Part model, mm, in its own coordinate system. A direction names the side the tool comes from. Round coordinates to 2 decimals unless told otherwise and drop trailing zeros. Loops run counter-clockwise (first coordinate to the right, second up) from the corner with the lowest first, then second, coordinate; pieces in that order, holes last.
1) Band-saw the part on A-A, the plane z = 30.5. Write the cut outline in (x, y), then the cut area to 3 significant figures.
2) Probe line 1 (Y direction, x = 13.5, z = 8.5); line 2 (X direction, y = 0, z = 29.7). List the from-to ranges inside material, lowest first.
3) Drop flat-ended pins along their axis: P1, Ø2, axis at x = 12, y = 3.5, coming from the -Z side; P2, Ø11.5, axis at x = 0, y = 0, coming from the -Z side; P3, Ø1.5, axis at x = -11.5, y = -6.5, coming from the +Z side; P4, Ø1.5, axis at x = -13.5, y = -0.5, coming from the +Z side. Give the stop position or say it passes through.
4) Mould opens along X. For faces 1 (the cylindrical face through (8.89, -16.01, 12.62)), 2 (the conical face through (8.17, -8.33, 32.24)), 3 (the flat face through (8, -7, 33.5)) say: +X half, -X half, draft (parallel to the pull), parting line (faces both ways), or undercut.
5) Band-saw the part on B-B, the plane y = 0. Write the cut outline in (x, z), then the cut area to 3 significant figures.
6) Band-saw the part on D-D, the plane z = 13. Write the cut outline in (x, y).
7) Band-saw the part on C-C, the plane z = 2. Write the cut outline in (x, y), then the cut area to 3 significant figures.
8) 3-axis set-ups, long thin cutter, end or side, ignore diameter. For faces 4 (the cylindrical face through (-7.406, -16.014, 13.875)), 5 (the cylindrical face through (8.21, 8.05, 30.99)), 6 (the cylindrical face through (8.05, -8.21, 30.99)): which of +Z, -Z, +X, -X, +Y, -Y reach the whole face in a straight line?
from build123d import *

# Parameters (mm, degrees)
F0_W      = 34
F0_H      = 34
F0_W_2    = 30
F0_H_2    = 30
F1_DEPTH  = 2
F2_DEPTH  = 28
F4_W      = 34
F4_H      = 34
F4_W_2    = 30
F4_H_2    = 30
F5_DEPTH  = 2
F9_DEPTH  = 3.5
F3_R      = 4.05
F3_R_2    = 1
F3_R_3    = 1.0373308001
F10_DEPTH = 2
F11_W     = 34
F11_H     = 34
F12_DEPTH = 2


with BuildPart() as f1:
    # F0 (on Top) → F1 (new body)
    with BuildSketch(Plane.XY):
        Rectangle(F0_W, F0_H)
        Rectangle(F0_W_2, F0_H_2, mode=Mode.SUBTRACT)
        Rectangle(F0_W_2, F0_H_2)
    extrude(amount=-F1_DEPTH)

    # F0 (on Top) → F2 (join)
    with BuildSketch(Plane.XY):
        Rectangle(F0_W, F0_H)
        Rectangle(F0_W_2, F0_H_2, mode=Mode.SUBTRACT)
    extrude(amount=F2_DEPTH)

    # F4 (on face) → F5 (join)
    with BuildSketch(Plane.XY.offset(28)):
        Rectangle(F4_W, F4_H)
        Rectangle(F4_W_2, F4_H_2, mode=Mode.SUBTRACT)
        Rectangle(F4_W_2, F4_H_2)
        with BuildLine():
            ThreePointArc((11.4562390281, 1.0022910416), (11.4890545482, 0.5016229547), (11.5, 0))
            ThreePointArc((11.5, 0), (11.4890545482, -0.5016229547), (11.4562390281, -1.0022910416))
            ThreePointArc((11.4562390281, -1.0022910416), (0, -11.5), (-11.4562390281, -1.0022910416))
            ThreePointArc((-11.4562390281, -1.0022910416), (-11.5, 0), (-11.4562390281, 1.0022910416))
            ThreePointArc((-11.4562390281, 1.0022910416), (0, 11.5), (11.4562390281, 1.0022910416))
        make_face(mode=Mode.SUBTRACT)
    extrude(amount=F5_DEPTH)

    # F6 (on Front) → F7 (revolve)
    with BuildSketch(Plane.XZ):
        Polygon((-11.5, 32), (-11.5, 30), (-9.5, 30), (-9.5, 33.5), (-12.5503113073, 33.5), align=None)
        Polygon((-9.5, 30), (-11.5, 30), (-11.5, 28), (-10.5, 28), (-9.5, 28), align=None)
    revolve(axis=Axis((0, 0, 27.9606003314), (0, 0, 1)))

    # F8 (on face) → F9 (cut)
    with BuildSketch(Plane.XY.offset(33.5)):
        with BuildLine():
            Line((9.4638496319, 0.8279795561), (0, 0))
            Line((0, 0), (9.4638496319, -0.8279795561))
            ThreePointArc((9.4638496319, -0.8279795561), (9.490958105, -0.41438418), (9.5, 0))
            ThreePointArc((9.5, 0), (9.490958105, 0.41438418), (9.4638496319, 0.8279795561))
        make_face()
        with BuildLine():
            Line((-9.4638496319, -0.8279795561), (0, 0))
            Line((0, 0), (-9.4638496319, 0.8279795561))
            ThreePointArc((-9.4638496319, 0.8279795561), (-9.5, 0), (-9.4638496319, -0.8279795561))
        make_face()
        with BuildLine():
            ThreePointArc((9.5, 0), (9.490958105, -0.41438418), (9.4638496319, -0.8279795561))
            Line((9.4638496319, -0.8279795561), (11.4562390281, -1.0022910416))
            Line((11.4562390281, -1.0022910416), (12.5025535837, -1.0938317037))
            ThreePointArc((12.5025535837, -1.0938317037), (12.5383661919, -0.5474368905), (12.5503113073, 0))
            ThreePointArc((12.5503113073, 0), (12.5383661919, 0.5474368905), (12.5025535837, 1.0938317037))
            Line((12.5025535837, 1.0938317037), (11.4562390281, 1.0022910416))
            Line((11.4562390281, 1.0022910416), (9.4638496319, 0.8279795561))
            ThreePointArc((9.4638496319, 0.8279795561), (9.490958105, 0.41438418), (9.5, 0))
        make_face()
        with BuildLine():
            Line((-11.4562390281, -1.0022910416), (-9.4638496319, -0.8279795561))
            ThreePointArc((-9.4638496319, -0.8279795561), (-9.5, 0), (-9.4638496319, 0.8279795561))
            Line((-9.4638496319, 0.8279795561), (-11.4562390281, 1.0022910416))
            Line((-11.4562390281, 1.0022910416), (-12.5025535837, 1.0938317037))
            ThreePointArc((-12.5025535837, 1.0938317037), (-12.5503113073, 0), (-12.5025535837, -1.0938317037))
            Line((-12.5025535837, -1.0938317037), (-11.4562390281, -1.0022910416))
        make_face()
        with BuildLine():
            Line((1.0938317037, -12.5025535837), (0.8279795561, -9.4638496319))
            ThreePointArc((0.8279795561, -9.4638496319), (0, -9.5), (-0.8279795561, -9.4638496319))
            Line((-0.8279795561, -9.4638496319), (-1.0938317037, -12.5025535837))
            ThreePointArc((-1.0938317037, -12.5025535837), (0, -12.5503113073), (1.0938317037, -12.5025535837))
        make_face()
        with BuildLine():
            Line((-1.0938317037, 12.5025535837), (-0.8279795561, 9.4638496319))
            ThreePointArc((-0.8279795561, 9.4638496319), (0, 9.5), (0.8279795561, 9.4638496319))
            Line((0.8279795561, 9.4638496319), (1.0938317037, 12.5025535837))
            ThreePointArc((1.0938317037, 12.5025535837), (0, 12.5503113073), (-1.0938317037, 12.5025535837))
        make_face()
    extrude(amount=-F9_DEPTH, mode=Mode.SUBTRACT)

    # F3 (on face) → F10 (cut, through all)
    with BuildSketch(Plane.XZ.offset(17)):
        with Locations((0, 13)):
            Circle(F3_R)
        with Locations((7.9639680702, 13)):
            Circle(F3_R_2)
        with Locations((-7.9639680702, 13)):
            Circle(F3_R_3)
    extrude(amount=-F10_DEPTH, mode=Mode.SUBTRACT)

    # F11 (on face) → F12 (cut)
    with BuildSketch(Plane(origin=(0, 0, -2), x_dir=(1, 0, 0), z_dir=(0, 0, -1))):
        Rectangle(F11_W, F11_H)
    extrude(amount=-F12_DEPTH, mode=Mode.SUBTRACT)


solid = f1.part
Reported:
1. outline: (-11.46, -1) arc R11.5 ccw to (-1, -11.46) - (-0.83, -9.46) arc R9.5 cw to (-9.46, -0.83) - close; (-11.46, 1) - (-9.46, 0.83) arc R9.5 cw to (-0.83, 9.46) - (-1, 11.46) arc R11.5 ccw to start; (0.83, -9.46) - (1, -11.46) arc R11.5 ccw to (11.46, -1) - (9.46, -0.83) arc R9.5 cw to start; (0.83, 9.46) arc R9.5 cw to (9.46, 0.83) - (11.46, 1) arc R11.5 ccw to (1, 11.46) - close
1. area: 117 mm2
2. line 1: y = -17 to -15, 15 to 17
2. line 2: x = -17 to -9.5, 9.5 to 17
3. P1: stops at z = 28
3. P2: passes through
3. P3: stops at z = 33.5
3. P4: stops at z = 30
4. face 1: undercut
4. face 2: +X half
4. face 3: draft
5. outline: (-17, 0) - (-15, 0) - (-15, 28) - (-9.5, 28) - (-9.5, 30) - (-17, 30) - close; (9.5, 28) - (15, 28) - (15, 0) - (17, 0) - (17, 30) - (9.5, 30) - close
5. area: 142 mm2
6. outline: (-17, -17) - (-9, -17) - (-9, -15) - (-15, -15) - (-15, 15) - (15, 15) - (15, -15) - (8.96, -15) - (8.96, -17) - (17, -17) - (17, 17) - (-17, 17) - close; (-6.93, -17) - (-4.05, -17) - (-4.05, -15) - (-6.93, -15) - close; (4.05, -17) - (6.96, -17) - (6.96, -15) - (4.05, -15) - close
7. outline: (-17, -17) - (17, -17) - (17, 17) - (-17, 17) - close; hole (-15, -15) - (15, -15) - (15, 15) - (-15, 15) - close
7. area: 256 mm2
8. face 4: -Y
8. face 5: +X, +Y
8. face 6: +X, -Y
